from build123d import *


with BuildPart() as part:
    # Sketch4 → Revolve1 (revolve)
    with BuildSketch(Plane(origin=(0, 0, 0), x_dir=(0, 0, -1), z_dir=(1, 0, 0))):
        Polygon((0, 25), (0, -25), (-31, -25), (-31, -11.639049179), (-57, -19.096481272), (-57, -21.096481272), (-67, -21.096481272), (-67, -16.096481272), (-42, -8.92587349), (-42, -3.225013879), (-67, 7.903518728), (-67, 12.903518728), (-57, 12.903518728), (-57, 10.903518728), (-31, -0.670155183), (-31, 5), (-27, 5), (-27, 25), align=None)
    revolve(axis=Axis((0, 25, 0), (0, -1, 0)))


solid = part.part
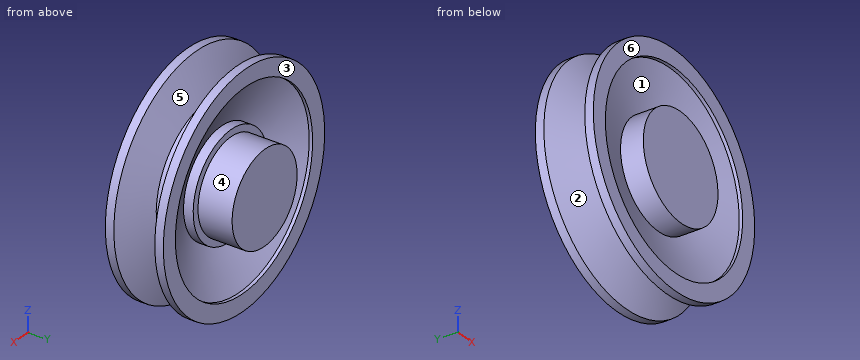
Model file for the job. Use its own axes, mm. Face numbers are marked on the shaded views. A direction names the side the tool comes from. Give positions to 0.01 mm unless a question says otherwise; leave off trailing zeros. Order: outer loops, then holes, each group sorted by start corner. A loop starts at its lowest first (then second) coordinate and runs counter-clockwise, first axis right, second up. Notation, with made-up numbers: (-6.75, 38) - (31.25, 38) arc R19 cw to (31.25, 70) - close; hole circle Ø5 at (12.5, 57.25). An arc over 180 degrees is marked (long way). One line per item, written item: value.
Item 1: Wall check: line 1 (X direction, y = 12, z = 0); line 2 (X direction, y = -20, z = 0). Give the ranges that are in metal, low to high.
Response values:
line 1: -67 to -57, -27 to 27, 57 to 67
line 2: -67 to -57, -31 to 31, 57 to 67
Item 2: Tool access for the marked faces 4, 5 and 6: list every direction of +Z, -Z, +X, -X, +Y, -Y with a clear straight run to the whole face (end or side of a thin tool).
Response values:
face 4: +Y
face 5: none
face 6: -Y
Item 3: Slice it at C-C (y = -7). List the corners of the cut face in (x, z), then the cut area to 3 significant figures.
Response values:
outline: circle Ø84 at (0, 0)
area: 5,540 mm2
Item 4: Two-plate mould, pull along Z, no slides. Class the marked faces 1, 2 and 3: released by +Z, released by -Z, zero draft, split by the parting line, or undercut.
Response values:
face 1: undercut
face 2: split by the parting line
face 3: zero draft
Item 5: Pin check, flat tips, straight feed: pin 1 Ø8 at (x, z) = (40, -22.5) entering from -Y; pin 2 Ø2 at (y, z) = (-15.5, -50) entering from -X; pin 3 Ø12 at (x, z) = (31.5, -49.5) entering from -Y. Stop position of each tip, or through.
Response values:
pin 1: y = -17.06
pin 2: x = -45.48
pin 3: y = -21.1
